```python
from build123d import *

# Parameters (mm, degrees)
SCHIZZO1_W                   = 4
SCHIZZO1_H                   = 4
SCHIZZO1_R                   = 1.5
SCHIZZO1_W_2                 = 30
SCHIZZO1_H_2                 = 12
ESTRUSIONE_ESTRUSIONE1_DEPTH = 1
SCHIZZO2_W                   = 29.5
SCHIZZO2_H                   = 11.5
ESTRUSIONE_ESTRUSIONE2_DEPTH = 8


with BuildPart() as part:
    # Schizzo1 → Estrusione-Estrusione1 (new body)
    # profile 1 of 3: a face of its own
    with BuildSketch(Plane.XY):
        with Locations((-2, 6)):
            Rectangle(SCHIZZO1_W, SCHIZZO1_H)
        with Locations((-2, 6)):
            Circle(SCHIZZO1_R, mode=Mode.SUBTRACT)
    # profile 2 of 3: a face of its own
    with BuildSketch(Plane.XY):
        with Locations((15, 6)):
            Rectangle(SCHIZZO1_W_2, SCHIZZO1_H_2)
    # profile 3 of 3: a face of its own
    with BuildSketch(Plane.XY):
        with Locations((32, 6)):
            Rectangle(SCHIZZO1_W, SCHIZZO1_H)
        with Locations((32, 6)):
            Circle(SCHIZZO1_R, mode=Mode.SUBTRACT)
    extrude(amount=ESTRUSIONE_ESTRUSIONE1_DEPTH)

    # Schizzo2 → Estrusione-Estrusione2 (add)
    with BuildSketch(Plane.XY.offset(1)):
        with Locations((15, 6)):
            Rectangle(SCHIZZO2_W, SCHIZZO2_H)
    extrude(amount=ESTRUSIONE_ESTRUSIONE2_DEPTH)


solid = part.part
```
Here's how the part is built. I have some questions about the finished solid (model axes, mm). A direction names the side the tool comes from. Give positions to 0.01 mm unless a question says otherwise; leave off trailing zeros. Loops run counter-clockwise (first coordinate to the right, second up) from the corner with the lowest first, then second, coordinate; pieces in that order, holes last. Notation, with made-up numbers: (21, 59) -> (40, 59) arc R28 ccw to (40, 85) -> close; hole circle Ø8 at (47.25, 29.25). An arc over 180 degrees is marked (long way). Use one line per item in the form item = value. Start each with the question number.
1) Imagine slicing it at A-A (y = 6). Please give me the cut outline in (x, z), then the cut area to 3 significant figures.
2) Imagine slicing it at B-B (x = 32). Please give me the cut outline in (y, z), then the cut area to 3 significant figures.
3) Imagine slicing it at C-C (z = 0.5). Please give me the cut outline in (x, y), then the cut area to 3 significant figures.
4) Please list where these lines run through material, in increasing order: line 1 along Y through (x, z) = (32, 0.6); line 2 along X through (y, z) = (1, 6.25); line 3 along Y through (x, z) = (29, 2.25).
5) Thinking about a two-plate mould opening in Y: for faces 1 (the face through (30.5, 6.07, 0.49)), 2 (the face through (29.75, 6, 5)), 3 (the face through (-2, 4, 0.5)), which applies, +Y half, -Y half, draft (parallel to the pull), parting line (faces both ways), or undercut?
6) Which directions (+Z, -Z, +X, -X, +Y, -Y) give clear straight access to the entire face, cutting with the end or side of a thin tool? Please do faces 4 (the face through (0, 2, 0.5)), 5 (the face through (30, 10, 0.5)), 6 (the face through (0, 10, 0.5)), 7 (the face through (0.25, 6, 5)).
7) Imagine slicing it at D-D (y = 8.5). Please give me the cut outline in (x, z).
8) For P1, Ø0.8, axis at y = 10.5, z = 0.5, coming from the +X side; P2, Ø5, axis at y = 4, z = 4.5, coming from the +X side; P3, Ø1.1, axis at x = 32, z = 0.5, coming from the +Y side; P4, Ø2.5, axis at x = 32, y = 6, coming from the +Z side, each with a flat end and sliding along its axis, tell me the tip position at first contact or that it passes through.
Check values:
q1.outline = (-4, 0) -> (-3.5, 0) -> (-3.5, 1) -> (-4, 1) -> close; (-0.5, 0) -> (30.5, 0) -> (30.5, 1) -> (29.75, 1) -> (29.75, 9) -> (0.25, 9) -> (0.25, 1) -> (-0.5, 1) -> close; (33.5, 0) -> (34, 0) -> (34, 1) -> (33.5, 1) -> close
q1.area = 268 mm^2
q2.outline = (4, 0) -> (4.5, 0) -> (4.5, 1) -> (4, 1) -> close; (7.5, 0) -> (8, 0) -> (8, 1) -> (7.5, 1) -> close
q2.area = 1.00 mm^2
q3.outline = (-4, 4) -> (0, 4) -> (0, 0) -> (30, 0) -> (30, 4) -> (34, 4) -> (34, 8) -> (30, 8) -> (30, 12) -> (0, 12) -> (0, 8) -> (-4, 8) -> close; hole circle Ø3 at (-2, 6); hole circle Ø3 at (32, 6)
q3.area = 378 mm^2
q4.line_1 = 4 to 4.5, 7.5 to 8
q4.line_2 = 0.25 to 29.75
q4.line_3 = 0.25 to 11.75
q5.face_1 = undercut
q5.face_2 = draft
q5.face_3 = -Y half
q6.face_4 = +Z, -Z, -X, -Y
q6.face_5 = +Z, -Z, +X, +Y
q6.face_6 = +Z, -Z, -X, +Y
q6.face_7 = +Z, -X, +Y, -Y
q7.outline = (0, 0) -> (30, 0) -> (30, 1) -> (29.75, 1) -> (29.75, 9) -> (0.25, 9) -> (0.25, 1) -> (0, 1) -> close
q8.P1 = 30
q8.P2 = 29.75
q8.P3 = 8
q8.P4 = through
